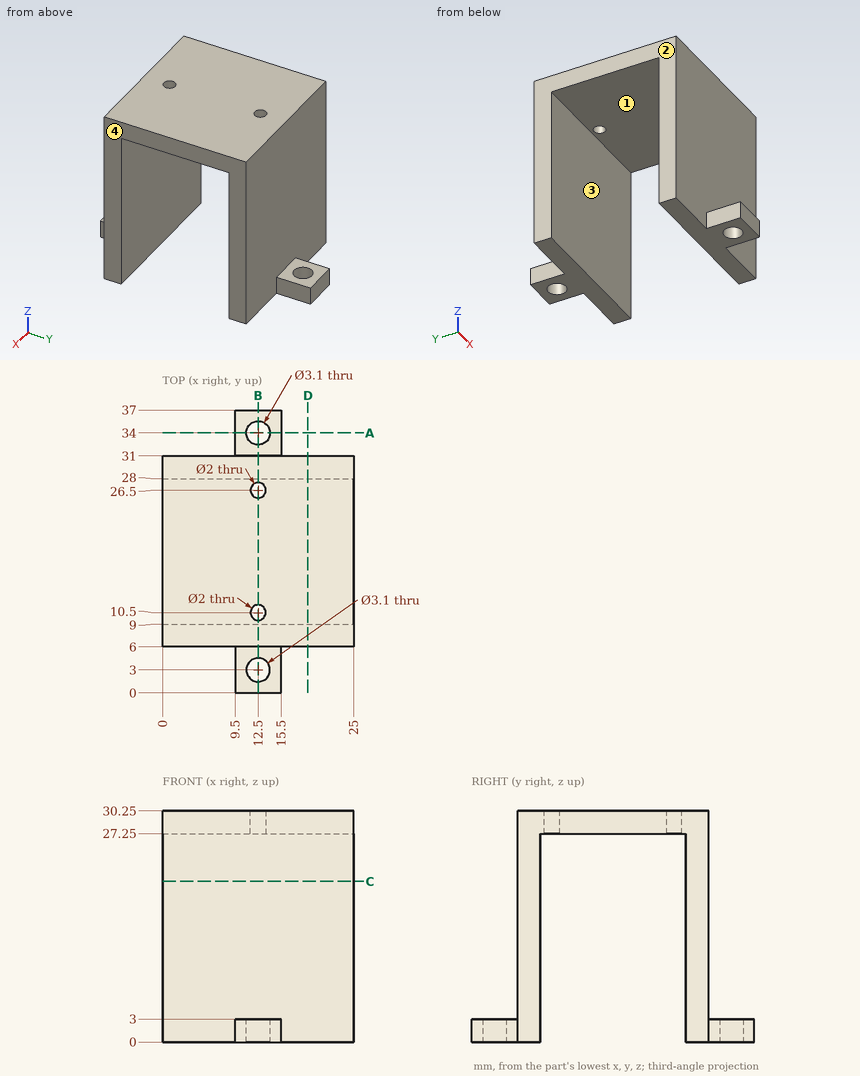
Geometry: see drawing. Coordinates: mm, zero at the bounding-box minimum. A direction names the side the tool comes from. Coordinates: 2 decimals unless noted, no trailing zeros. Loops run counter-clockwise (first coordinate to the right, second up) from the corner with the lowest first, then second, coordinate; pieces in that order, holes last.
(1) Set-up query: the marked faces 3 and 4. Return all of +Z, -Z, +X, -X, +Y, -Y with unobstructed straight access to the full face (end or side cutting, diameter ignored); none if empty.
(2) First-contact query: pin 1 Ø12.5 at (x, z) = (11.5, 13) entering from -Y; pin 2 Ø0.9 at (y, z) = (35.5, 2) entering from -X; pin 3 Ø1 at (x, y) = (15, 15.5) entering from -Z; pin 4 Ø1.8 at (x, y) = (12.5, 26.5) entering from -Z. Flat tips, straight axial feed; report the tip coordinate or a pass-through.
(3) Material intervals for probe 1 along Y at (x, z) = (12.5, 2.4); probe 2 along Y at (x, z) = (12.5, 29); probe 3 along Y at (x, z) = (1.5, 27), sorted ascending.
(4) Section A-A on y = 34. Return the cut outline in (x, z).
(5) Pull-direction query (Y, two-part tool) for the marked faces 1 and 2; classes: released by +Y, released by -Y, zero draft, split by the parting line, or undercut.
(6) Section D-D on x = 19. Return the cut outline in (y, z), then the cut area to 4 significant figures.
(7) Section C-C on z = 21. Return the cut outline in (x, y).
(8) Section B-B on x = 12.5. Return the cut outline in (y, z), then the cut area to 3 significant figures.
Data:
1. face 3: -Z, +X, -X
1. face 4: +Z, -Z, +X, +Y, -Y
2. pin 1: stops at y = 6
2. pin 2: stops at x = 9.5
2. pin 3: stops at z = 27.25
2. pin 4: passes through
3. probe 1: y = 0 to 1.45, 4.55 to 9, 28 to 32.45, 35.55 to 37
3. probe 2: y = 6 to 9.5, 11.5 to 25.5, 27.5 to 31
3. probe 3: y = 6 to 9, 28 to 31
4. outline: (9.5, 0) - (10.95, 0) - (10.95, 3) - (9.5, 3) - close; (14.05, 0) - (15.5, 0) - (15.5, 3) - (14.05, 3) - close
5. face 1: undercut
5. face 2: zero draft
6. outline: (6, 0) - (9, 0) - (9, 27.25) - (28, 27.25) - (28, 0) - (31, 0) - (31, 30.25) - (6, 30.25) - close
6. area: 238.5 mm2
7. outline: (0, 6) - (25, 6) - (25, 9) - (0, 9) - close; (0, 28) - (25, 28) - (25, 31) - (0, 31) - close
8. outline: (0, 0) - (1.45, 0) - (1.45, 3) - (0, 3) - close; (4.55, 0) - (9, 0) - (9, 27.25) - (9.5, 27.25) - (9.5, 30.25) - (6, 30.25) - (6, 3) - (4.55, 3) - close; (11.5, 27.25) - (25.5, 27.25) - (25.5, 30.25) - (11.5, 30.25) - close; (27.5, 27.25) - (28, 27.25) - (28, 0) - (32.45, 0) - (32.45, 3) - (31, 3) - (31, 30.25) - (27.5, 30.25) - close; (35.55, 0) - (37, 0) - (37, 3) - (35.55, 3) - close
8. area: 244 mm2
